For this review, take the finished solid that the model builds, in its own axes (mm). A direction names the side the tool comes from. Round coordinates to 2 decimals unless told otherwise and drop trailing zeros. Loops run counter-clockwise (first coordinate to the right, second up) from the corner with the lowest first, then second, coordinate; pieces in that order, holes last.
1) Insertion check: pin 1 (4 mm diameter, centred on x = 3, y = -6.5, fed in from -Z); pin 2 (1.5 mm diameter, centred on y = -4.5, z = 4, fed in from -X); pin 3 (0.6 mm diameter, centred on x = -4.5, y = -7, fed in from +Z). Each pin has a flat end and moves straight along its axis. Give the tip position at first contact, or say it passes through.
2) Take a section at B-B (y = -2.5). State the section outline as (x, z) points.
3) Take a section at C-C (z = -19.5). State the section outline as (x, y) points.
4) Take a section at D-D (x = 15). State the section outline as (y, z) points.
5) Tool access review of faces 5 (the flat face through (0, -5, 4)), 6 (the flat face through (7.98, -4.93, -20.85)), 7 (the flat face through (17.53, -4.93, -20.52)): name each direction out of +Z, -Z, +X, -X, +Y, -Y from which nothing blocks a thin tool from reaching the whole face with its end or side.
6) Wall thickness on L1, parallel to X at y = -7, z = -12; L2, parallel to Z at x = 9, y = -0.25; L3, parallel to Z at x = 22.5, y = -4.25: over which ranges is each line inside the solid? List them lowest first.
7) Take a section at A-A (x = 9). State the section outline as (y, z) points.
8) Mouldability with a two-part tool opening along X and no side actions: class faces 1 (the flat face through (11, -10, -13)), 2 (the flat face through (6.082, -4.93, -26.406)), 3 (the flat face through (20.08, -4.93, -11.35)), 4 (the flat face through (10.599, -4.93, -8.145)) as pulls with the +X half, pulls with the -X half, needs draft (parallel to the pull), parting line crosses it, or undercut.
```python
from build123d import *

# Parameters (mm, degrees)
F1_DEPTH = 10


with BuildPart() as f1:
    # F0 (on Front) → F1 (new body)
    with BuildSketch(Plane.XZ):
        with BuildLine():
            ThreePointArc((2.028823, -2.343902), (-1.288536, -2.819517), (-3.1, 0))
            Line((-3.1, 0), (-4.1, 0))
            Line((-4.1, 0), (-5, 0))
            ThreePointArc((-5, 0), (-3.266365, -3.785612), (0.732343, -4.946077))
            Line((0.732343, -4.946077), (11.706972, -17.625082))
            Line((11.706972, -17.625082), (4.145997, -24.169672))
            Line((4.145997, -24.169672), (8.072751, -28.706257))
            Line((8.072751, -28.706257), (27.252344, -12.104882))
            Line((27.252344, -12.104882), (23.807724, -8.125308))
            Line((23.807724, -8.125308), (16.246749, -14.669898))
            Line((16.246749, -14.669898), (4.789988, -1.433882))
            ThreePointArc((4.789988, -1.433882), (4.010574, 2.985849), (0, 5))
            Line((0, 5), (0, 4.1))
            Line((0, 4.1), (0, 3.1))
            ThreePointArc((0, 3.1), (2.904832, 1.082567), (2.028823, -2.343902))
        make_face()
    extrude(amount=F1_DEPTH)


solid = f1.part
```
Response:
1. pin 1: stops at z = -25.16
1. pin 2: stops at x = 0
1. pin 3: stops at z = 0
2. outline: (-5, 0) arc R5 ccw to (0.73, -4.95) - (11.71, -17.63) - (4.15, -24.17) - (8.07, -28.71) - (27.25, -12.1) - (23.81, -8.13) - (16.25, -14.67) - (4.79, -1.43) arc R5 ccw to (0, 5) - (0, 3.1) arc R3.1 cw (long way) to (-3.1, 0) - close
3. outline: (9.54, -10) - (18.71, -10) - (18.71, 0) - (9.54, 0) - close
4. outline: (-10, -22.71) - (0, -22.71) - (0, -13.23) - (-10, -13.23) - close
5. face 5: +Z, -X, +Y, -Y
5. face 6: -X, +Y, -Y
5. face 7: -Z, +X, +Y, -Y
6. L1: x = 6.84 to 13.94, 19.33 to 27.16
6. L2: z = -27.9 to -19.97, -14.5 to -6.3
6. L3: z = -16.22 to -9.26
7. outline: (-10, -27.9) - (0, -27.9) - (0, -19.97) - (-10, -19.97) - close; (-10, -14.5) - (0, -14.5) - (0, -6.3) - (-10, -6.3) - close
8. face 1: needs draft
8. face 2: pulls with the -X half
8. face 3: undercut
8. face 4: undercut
